from build123d import *

# Parameters (mm, degrees)
SKETCH_1_R          = 1.5
EXTRUDE_1_DEPTH     = 3
SKETCH_2_W          = 70
SKETCH_2_H          = 22
EXTRUDE_2_DEPTH     = 3
SKETCH_3_W          = 20
SKETCH_3_H          = 21.549001307
CUT_EXTRUDE_1_DEPTH = 3
SKETCH_4_W          = 1
SKETCH_4_H          = 2
EXTRUDE_3_DEPTH     = 5
SKETCH_5_W          = 40
SKETCH_5_H          = 25
EXTRUDE_4_DEPTH     = 3
SKETCH_6_W          = 79.808748454
SKETCH_6_H          = 4
CUT_EXTRUDE_2_DEPTH = 5
SKETCH_7_W          = 5
SKETCH_7_H          = 25
EXTRUDE_5_DEPTH     = 30
SKETCH_8_R          = 2.75
SKETCH_8_R_2        = 1.6
CUT_EXTRUDE_3_DEPTH = 5
SKETCH_9_W          = 5
SKETCH_9_H          = 25
EXTRUDE_6_DEPTH     = 3
SKETCH_10_W         = 7
SKETCH_10_H         = 39.176748617
CUT_EXTRUDE_4_DEPTH = 53.490475326


with BuildPart() as part:
    # 草图1 → 凸台-拉伸1 (new body)
    # profile 1 of 2: a face of its own
    with BuildSketch(Plane.XY):
        Polygon((26, -22.5), (35, -22.5), (35, 22.5), (12.5, 22.5), (12.5, -7.5), (-12.5, -7.5), (-12.5, 22.5), (-35, 22.5), (-35, -22.5), (-26, -22.5), (-26, -15), (26, -15), align=None)
        with Locations((-30.4, -17.95)):
            Circle(SKETCH_1_R, mode=Mode.SUBTRACT)
        with Locations((30.4, -17.95)):
            Circle(SKETCH_1_R, mode=Mode.SUBTRACT)
        with Locations((-30.4, 17.95)):
            Circle(SKETCH_1_R, mode=Mode.SUBTRACT)
        with Locations((30.4, 17.95)):
            Circle(SKETCH_1_R, mode=Mode.SUBTRACT)
    # profile 2 of 2: a face of its own
    with BuildSketch(Plane.XY):
        Polygon((12.5, 22.5), (35, 22.5), (35, 24.5), (-35, 24.5), (-35, 22.5), (-12.5, 22.5), align=None)
    extrude(amount=EXTRUDE_1_DEPTH)

    # 草图2 → 凸台-拉伸2 (add)
    with BuildSketch(Plane(origin=(0, 24.5, 0), x_dir=(1, 0, 0), z_dir=(0, 1, 0))):
        with Locations((0, 8)):
            Rectangle(SKETCH_2_W, SKETCH_2_H)
    extrude(amount=EXTRUDE_2_DEPTH)

    # 草图3 → 切除-拉伸1 (cut)
    with BuildSketch(Plane(origin=(0, 27.5, 0), x_dir=(1, 0, 0), z_dir=(0, 1, 0))):
        with Locations((18, 14.774500654)):
            Rectangle(SKETCH_3_W, SKETCH_3_H)
    extrude(amount=-CUT_EXTRUDE_1_DEPTH, mode=Mode.SUBTRACT)

    # 草图4 → 凸台-拉伸3 (add)
    with BuildSketch(Plane.XY.offset(3)):
        with Locations((4.5, 28.5)):
            Rectangle(SKETCH_4_W, SKETCH_4_H)
        with Locations((-4.5, 28.5)):
            Rectangle(SKETCH_4_W, SKETCH_4_H)
    extrude(amount=-EXTRUDE_3_DEPTH)

    # 草图5 → 凸台-拉伸4 (add)
    with BuildSketch(Plane(origin=(0, 27.5, 0), x_dir=(1, 0, 0), z_dir=(0, 1, 0))):
        with Locations((-25, 2.5)):
            Rectangle(SKETCH_5_W, SKETCH_5_H)
    extrude(amount=EXTRUDE_4_DEPTH)

    # 草图6 → 切除-拉伸2 (cut)
    with BuildSketch(Plane(origin=(0, 27.5, 0), x_dir=(1, 0, 0), z_dir=(0, 1, 0))):
        with Locations((4.904374227, 17)):
            Rectangle(SKETCH_6_W, SKETCH_6_H)
    extrude(amount=-CUT_EXTRUDE_2_DEPTH, mode=Mode.SUBTRACT)

    # 草图7 → 凸台-拉伸5 (add)
    with BuildSketch(Plane(origin=(0, 30.5, 0), x_dir=(1, 0, 0), z_dir=(0, 1, 0))):
        with Locations((-42.5, 2.5)):
            Rectangle(SKETCH_7_W, SKETCH_7_H)
    extrude(amount=-EXTRUDE_5_DEPTH)

    # 草图8 → 切除-拉伸3 (cut)
    with BuildSketch(Plane.ZY.offset(45)):
        with Locations((-2.5, 10.5)):
            Circle(SKETCH_8_R)
        with Locations((-2.5, 18.5)):
            Circle(SKETCH_8_R_2)
        with Locations((5.5, 10.5)):
            Circle(SKETCH_8_R_2)
        with Locations((-2.5, 2.5)):
            Circle(SKETCH_8_R_2)
        with Locations((-10.5, 10.5)):
            Circle(SKETCH_8_R_2)
    extrude(amount=-CUT_EXTRUDE_3_DEPTH, mode=Mode.SUBTRACT)

    # 草图9 → 凸台-拉伸6 (add)
    with BuildSketch(Plane.XZ.offset(-27.5)):
        with Locations((-37.5, -2.5)):
            Rectangle(SKETCH_9_W, SKETCH_9_H)
    extrude(amount=EXTRUDE_6_DEPTH)

    # 草图10 → 切除-拉伸4 (cut, through all)
    with BuildSketch(Plane(origin=(-5, 0, 0), x_dir=(0, 0, -1), z_dir=(1, 0, 0))):
        with Locations((-6.5, 10.911625692)):
            Rectangle(SKETCH_10_W, SKETCH_10_H)
    extrude(amount=-CUT_EXTRUDE_4_DEPTH, mode=Mode.SUBTRACT)


solid = part.part
Verification items for the finished model (mm, model axes). A direction names the side the tool comes from. Round coordinates to 2 decimals unless told otherwise and drop trailing zeros. Loops run counter-clockwise (first coordinate to the right, second up) from the corner with the lowest first, then second, coordinate; pieces in that order, holes last. Notation, with made-up numbers: (12, 49.25) - (61, 49.25) arc R18 cw to (61, 54.25) - close; hole circle Ø3 at (42.25, 28). An arc over 180 degrees is marked (long way). Use a Markdown table: item, result. Add a question column.
1. Section check A-A, the plane x = 30.4. Record the boundary of the cut face in (y, z).
2. Release check for a two-part mould opening along Y. For faces 1 (the face through (-13, 4, 3)), 2 (the face through (-25, 30.5, -6)), 3 (the face through (0, 22.5, 1)) record: released by +Y, released by -Y, zero draft, split by the parting line, or undercut.
3. Gauge pin test, flat ends, axial feed: pin 1 (2 mm diameter, centred on y = 28, z = 1.5, fed in from +X); pin 2 (5.5 mm diameter, centred on x = -8, z = -10.5, fed in from -Y); pin 3 (1.5 mm diameter, centred on x = 12.5, z = 2, fed in from -Y); pin 4 (4 mm diameter, centred on x = 25, z = -3.5, fed in from +Y). Record the tip position at first contact, or that the pin passes through.
4. Section check C-C, the plane y = 5. Record the boundary of the cut face in (x, z).
5. Access from +Z, -Z, +X, -X, +Y, -Y to the whole of each face (thin tool, end or side, straight path). Record for faces 4 (the face through (28, 26, -9)), 5 (the face through (-35, 1, 2)), 6 (the face through (-42.535, 13.227, -2.858)), 7 (the face through (-12.5, 7, 1)).
6. Section check B-B, the plane z = -10.5. Record the boundary of the cut face in (x, y).
7. Section check D-D, the plane z = -6.5. Record the boundary of the cut face in (x, y).
8. Thickness scan on probe 1 along Y at (x, z) = (-41.8, -2.5); probe 2 along X at (y, z) = (-18, 1); probe 3 along Y at (x, z) = (-1.5, 1.75). Record the ranges inside material, lowest first. Write a range as [from, to].
Checks:
| question | item | result |
|---|---|---|
| 1 | outline | (-22.5, 0) - (-19.45, 0) - (-19.45, 3) - (-22.5, 3) - close; (-16.45, 0) - (16.45, 0) - (16.45, 3) - (-16.45, 3) - close; (19.45, 0) - (24.5, 0) - (24.5, -15) - (27.5, -15) - (27.5, 3) - (19.45, 3) - close |
| 2 | face 1 | zero draft |
| 2 | face 2 | released by +Y |
| 2 | face 3 | undercut |
| 3 | pin 1 | stops at x = 35 |
| 3 | pin 2 | stops at y = 24.5 |
| 3 | pin 3 | stops at y = -15 |
| 3 | pin 4 | stops at y = 27.5 |
| 4 | outline | (-45, -15) - (-40, -15) - (-40, 3) - (-45, 3) - close; (-35, 0) - (-12.5, 0) - (-12.5, 3) - (-35, 3) - close; (12.5, 0) - (35, 0) - (35, 3) - (12.5, 3) - close |
| 5 | face 4 | -Z, +Y, -Y |
| 5 | face 5 | +Z, -Z, -Y |
| 5 | face 6 | -X |
| 5 | face 7 | +Z, -Z |
| 6 | outline | (-45, 0.5) - (-40, 0.5) - (-40, 8.9) - (-45, 8.9) - close; (-45, 12.1) - (-40, 12.1) - (-40, 24.5) - (8, 24.5) - (8, 27.5) - (-5, 27.5) - (-5, 30.5) - (-45, 30.5) - close; (28, 24.5) - (35, 24.5) - (35, 27.5) - (28, 27.5) - close |
| 7 | outline | (-45, 0.5) - (-40, 0.5) - (-40, 24.5) - (8, 24.5) - (8, 27.5) - (-5, 27.5) - (-5, 30.5) - (-45, 30.5) - close; (28, 24.5) - (35, 24.5) - (35, 27.5) - (28, 27.5) - close |
| 8 | probe 1 | y = [0.5, 0.9], [4.1, 7.75], [13.25, 16.9], [20.1, 30.5] |
| 8 | probe 2 | x = [-35, -31.9], [-28.9, -26], [26, 28.9], [31.9, 35] |
| 8 | probe 3 | y = [-15, -7.5], [22.5, 27.5] |
